Input: part model. Units: mm. Frame: model coordinates. A direction names the side the tool comes from. Round coordinates to 2 decimals unless told otherwise and drop trailing zeros. Order: outer loops, then holes, each group sorted by start corner. A loop starts at its lowest first (then second) coordinate and runs counter-clockwise, first axis right, second up.
Item 1: Cut plane D-D on x = -27.5. Output: boundary loops of the cut face in (y, z).
Item 2: First-contact query: pin 1 (3 mm diameter, centred on x = -53.51, z = -83.32, fed in from +Y); pin 2 (1 mm diameter, centred on y = 2.5, z = -26.5, fed in from -X). Flat tips, straight axial feed; report the tip coordinate or a pass-through.
Item 3: Cut plane A-A on z = 43. Output: boundary loops of the cut face in (x, y).
Item 4: Mould query, pull axis X, two halves, no side actions, for faces 1 (the flat face through (2, 3, 1)), 2 (the cylindrical face through (-71.4, 1.48, -7.28)), 3 (the flat face through (26.57, 1.48, -48.63)), 4 (the flat face through (-28.828, 1.479, 47.327)). Classes: released by +X, released by -X, zero draft, split by the parting line, or undercut.
Item 5: Line query: L1, parallel to Z at x = -8, y = 0.2; L2, parallel to Z at x = 28.5, y = 0.5; L3, parallel to X at y = 0.3, z = 4. Output: solid intervals per line, ascending.
Item 6: Cut plane B-B on y = 1.15. Output: boundary loops of the cut face in (x, z).
Item 7: Cut plane C-C on x = 46.5. Output: boundary loops of the cut face in (y, z).
Item 8: Reachability of faces 5 (the cylindrical face through (-19.515, 1.479, 35.449)), 6 (the flat face through (2, 0, 1)) from +Z, -Z, +X, -X, +Y, -Y: full face, straight path, thin tool, end or side. Return the list, or none.
Autodesk Inventor part; units mm, degrees
ref_plane "YZ Plane" through (0, 0, 0) normal (1, 0, 0) x (0, 1, 0)
ref_plane "XZ Plane" through (0, 0, 0) normal (0, 1, 0) x (-1, 0, 0)
ref_plane "XY Plane" through (0, 0, 0) normal (0, 0, 1) x (1, 0, 0)
sketch "Sketch1" plane through (0, 0, 0) normal (0, 1, 0) x (-1, 0, 0)
  circle A0 centre (98.9102, -4.6824) radius 1.6
  circle A1 centre (53.5102, -83.3176) radius 1.6
  circle A2 centre (-98.9102, 4.6824) radius 1.6
  circle A3 centre (-53.5102, 83.3176) radius 1.6
  line L0 (107.5705, -9.6824) -> (62.1705, -88.3176)
  line L1 (-62.1705, 88.3176) -> (-107.5705, 9.6824)
  line L2 (107.5705, -9.6824) -> (112.5705, -1.0222)
  line L3 (112.5705, -1.0222) -> (-57.1705, 96.9778)
  line L4 (112.5705, -1.0222) -> (308.5705, -1.0222) construction
  line L5 (-57.1705, 96.9778) -> (-62.1705, 88.3176)
  line L6 (62.1705, -88.3176) -> (57.1705, -96.9778)
  line L7 (57.1705, -96.9778) -> (-112.5705, 1.0222)
  line L8 (-112.5705, 1.0222) -> (-107.5705, 9.6824)
  line L9 (-15, -25.9808) -> (43, -25.9808) construction
  arc A4 (69.6208, 3.0607) -> (-32.1598, 61.8238) centre (-268.5566, -465.1538) ccw
  arc A5 (60.8381, -9.0992) -> (-38.2992, 48.1377) centre (-268.5566, -465.1538) ccw
  arc A6 (60.8381, -9.0992) -> (69.6208, 3.0607) centre (65.2295, -3.0192) ccw
  arc A7 (-32.1598, 61.8238) -> (-38.2992, 48.1377) centre (-35.2295, 54.9808) ccw
  arc A8 (69.6208, 3.0607) -> (-32.1598, 61.8238) centre (-268.5566, -465.1538) ccw
  arc A9 (60.8381, -9.0992) -> (-38.2992, 48.1377) centre (-268.5566, -465.1538) ccw
  arc A10 (-32.1598, 61.8238) -> (-38.2992, 48.1377) centre (-35.2295, 54.9808) ccw
  arc A11 (60.8381, -9.0992) -> (69.6208, 3.0607) centre (65.2295, -3.0192) ccw
  arc A12 (-69.6208, -3.0607) -> (32.1598, -61.8238) centre (268.5566, 465.1538) ccw
  arc A13 (-60.8381, 9.0992) -> (38.2992, -48.1377) centre (268.5566, 465.1538) ccw
  arc A14 (-60.8381, 9.0992) -> (-69.6208, -3.0607) centre (-65.2295, 3.0192) ccw
  arc A15 (32.1598, -61.8238) -> (38.2992, -48.1377) centre (35.2295, -54.9808) ccw
  point P0 (-50, -7)
  point P1 (-50, -17)
  point P2 (31.0622, -39.8013)
  point P3 (39.7224, -34.8013)
  point P4 (-31.0622, 39.8013)
  point P5 (-39.7224, 34.8013)
  point P6 (50, 7)
  point P7 (50, 17)
  point P8 (18.9378, 46.8013)
  point P9 (10.2776, 51.8013)
  point P10 (-18.9378, -46.8013)
  point P11 (-10.2776, -51.8013)
  point P12 (32.1598, -61.8238)
  dimension "d116" = 10
  dimension "d117" = 10
  dimension "d119" = 150
  dimension "d121" = 90
  dimension "d134" = 15
extrude "Extrusion5" add sketch "Sketch1" along normal blind 3
fillet "Fillet4" radius 5 4 edges at (57.1705, 1.5, 96.9778) (112.5705, 1.5, 1.0222) (-112.5705, 1.5, -1.0222) (-57.1705, 1.5, -96.9778)
properties part number "Tempat Batere"
From the geometry:
1. outline: (0, -79.85) - (3, -79.85) - (3, -59.71) - (0, -59.71) - close; (0, -43.16) - (3, -43.16) - (3, 13.22) - (0, 13.22) - close; (0, 30.77) - (3, 30.77) - (3, 48.09) - (0, 48.09) - close
2. pin 1: passes through
2. pin 2: stops at x = -98.15
3. outline: (-36.32, 0) - (-5.98, 0) - (-5.98, 3) - (-36.32, 3) - close; (27.17, 0) - (88.33, 0) - (88.33, 3) - (27.17, 3) - close
4. face 1: zero draft
4. face 2: undercut
4. face 3: released by +X
4. face 4: released by -X
5. L1: z = -68.59 to -50.31, -33.44 to 24.75, 41.9 to 59.35
5. L2: z = -47.52 to -30.17, -12.6 to 43.63, 60.17 to 80.42
5. L3: x = -103.87 to -68.32, -41.9 to 53.66, 72.67 to 97.46, 100.36 to 110.61
6. outline: (-110.07, -5.35) - (-107.57, -9.68) - (-62.17, -88.32) - (-59.67, -92.65) arc R5 ccw to (-52.84, -94.48) - (108.24, -1.48) arc R5 ccw to (110.07, 5.35) - (107.57, 9.68) - (62.17, 88.32) - (59.67, 92.65) arc R5 ccw to (52.84, 94.48) - (-108.24, 1.48) arc R5 ccw to start; hole circle Ø3.2 at (-98.91, -4.68); hole (-69.62, 3.06) arc R7.5 ccw to (-60.84, -9.1) arc R562.57 cw to (38.3, 48.14) arc R7.5 ccw to (32.16, 61.82) arc R577.58 ccw to start; hole circle Ø3.2 at (-53.51, -83.32); hole (-38.3, -48.14) arc R7.5 ccw to (-32.16, -61.82) arc R577.58 ccw to (69.62, -3.06) arc R7.5 ccw to (60.84, 9.1) arc R562.57 cw to start; hole circle Ø3.2 at (53.51, 83.32); hole circle Ø3.2 at (98.91, 4.68)
7. outline: (0, -37.12) - (3, -37.12) - (3, -18.92) - (0, -18.92) - close; (0, -0.92) - (3, -0.92) - (3, 90.82) - (0, 90.82) - close
8. face 5: +Y, -Y
8. face 6: +Z, -Z, +X, -X, -Y
